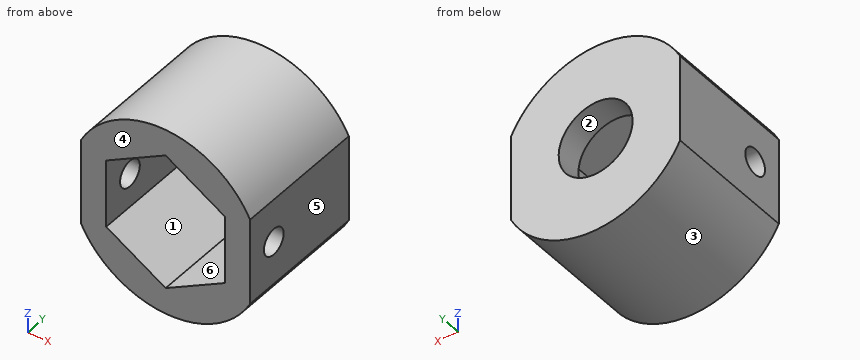
from build123d import *

# Parameters (mm, degrees)
ESBO_O9_R                   = 9
RESSALTO_EXTRUS_O1_DEPTH    = 12.5
ESBO_O12_R                  = 3.5
CORTE_EXTRUS_O9_DEPTH       = 18.839562775
CORTE_EXTRUS_O10_DEPTH      = 10
CORTE_EXTRUS_O11_DEPTH      = 18.839562775
CORTE_EXTRUS_O11_DEPTH_BACK = 18.839562775
ESBO_O14_R                  = 1.25
CORTE_EXTRUS_O12_DEPTH      = 18.83956296


with BuildPart() as part:
    # Esboço9 → Ressalto-extrusão1 (new body)
    with BuildSketch(Plane(origin=(0, 0, 0), x_dir=(1, 0, 0), z_dir=(0, 1, 0))):
        with Locations(Location((0, 0, 0), (0, 0, 270))):
            Circle(ESBO_O9_R)
    extrude(amount=RESSALTO_EXTRUS_O1_DEPTH)

    # Esboço12 → Corte-extrusão9 (cut, through all)
    with BuildSketch(Plane(origin=(0, 12.5, 0), x_dir=(1, 0, 0), z_dir=(0, 1, 0))):
        with Locations(Location((0, 0, 0), (0, 0, 270))):
            Circle(ESBO_O12_R)
    extrude(amount=-CORTE_EXTRUS_O9_DEPTH, mode=Mode.SUBTRACT)

    # Esboço13 → Corte-extrusão10 (cut)
    with BuildSketch(Plane.XZ):
        Polygon((0, 6.495190528), (-5.625, 3.247595264), (-5.625, -3.247595264), (0, -6.495190528), (5.625, -3.247595264), (5.625, 3.247595264), align=None)
    extrude(amount=-CORTE_EXTRUS_O10_DEPTH, mode=Mode.SUBTRACT)

    # Esboço14 → Corte-extrusão11 (cut, two sides: drawn at the far end of the back side and taken through both)
    with BuildSketch(Plane(origin=(0, 0, 0), x_dir=(0, 0, -1), z_dir=(1, 0, 0)).offset(-CORTE_EXTRUS_O11_DEPTH_BACK)):
        with Locations(Location((0, 3, 0), (0, 0, 270))):
            Circle(ESBO_O14_R)
    extrude(amount=CORTE_EXTRUS_O11_DEPTH + CORTE_EXTRUS_O11_DEPTH_BACK, mode=Mode.SUBTRACT)

    # Esboço15 → Corte-extrusão12 (cut, through all)
    with BuildSketch(Plane.XZ):
        with BuildLine():
            Line((-8, 4.123105626), (-8, -4.123105626))
            ThreePointArc((-8, -4.123105626), (-9, 0), (-8, 4.123105626))
        make_face()
        with BuildLine():
            Line((8, 4.123105626), (8, -4.123105626))
            ThreePointArc((8, -4.123105626), (9, 0), (8, 4.123105626))
        make_face()
    extrude(amount=-CORTE_EXTRUS_O12_DEPTH, mode=Mode.SUBTRACT)


solid = part.part
Model file for the job. Use its own axes, mm. Face numbers are marked on the shaded views. A direction names the side the tool comes from. Round coordinates to 2 decimals unless told otherwise and drop trailing zeros. Loops run counter-clockwise (first coordinate to the right, second up) from the corner with the lowest first, then second, coordinate; pieces in that order, holes last. Notation, with made-up numbers: (15.5, 29) - (48.5, 29) arc R18 cw to (48.5, 62) - close; hole circle Ø7 at (-22.75, -6.75). An arc over 180 degrees is marked (long way). Write each question's results on one line, items separated by ' | '.
(1) Saw through at C-C, the plane x = -1. List the corners of the cut face in (y, z), then the cut area to 3 significant figures.
Answer below:
outline: (0, -8.94) - (12.5, -8.94) - (12.5, -3.35) - (10, -3.35) - (10, -5.92) - (0, -5.92) - close; (0, 5.92) - (10, 5.92) - (10, 3.35) - (12.5, 3.35) - (12.5, 8.94) - (0, 8.94) - close | area: 88.5 mm^2
(2) 3-axis set-ups, long thin cutter, end or side, ignore diameter. For the marked faces 1 and 2: which of +Z, -Z, +X, -X, +Y, -Y reach the whole face in a straight line?
Answer below:
face 1: -Y | face 2: +Y, -Y
(3) Mould opens along X. For the marked faces 3, 4, 5 and 6 say: released by +X, released by -X, zero draft, split by the parting line, or undercut.
Answer below:
face 3: split by the parting line | face 4: zero draft | face 5: released by +X | face 6: undercut
(4) Saw through at D-D, the plane y = 9.25. List the corners of the cut face in (x, z) (3 decimals), then the cut area to 3 significant figures.
Answer below:
outline: (-8, -4.123) arc R9 ccw to (8, -4.123) - (8, 4.123) arc R9 ccw to (-8, 4.123) - close; hole (-5.625, -3.248) - (0, -6.495) - (5.625, -3.248) - (5.625, 3.248) - (0, 6.495) - (-5.625, 3.248) - close | area: 134 mm^2
(5) Saw through at B-B, the plane y = 3.75. List the corners of the cut face in (x, z) (3 decimals).
Answer below:
outline: (-8, -4.123) arc R9 ccw to (8, -4.123) - (8, -1) - (5.625, -1) - (5.625, -3.248) - (0, -6.495) - (-5.625, -3.248) - (-5.625, -1) - (-8, -1) - close; (-8, 1) - (-5.625, 1) - (-5.625, 3.248) - (0, 6.495) - (5.625, 3.248) - (5.625, 1) - (8, 1) - (8, 4.123) arc R9 ccw to (-8, 4.123) - close
(6) Pin check, flat tips, straight feed: pin 1 (2 mm diameter, centred on y = 3, z = 0, fed in from -X); pin 2 (5 mm diameter, centred on x = 0.5, y = 3.5, fed in from -Z); pin 3 (6 mm diameter, centred on x = -4.5, y = 10.5, fed in from +Z). Stop position of each tip, or through.
Answer below:
pin 1: passes through | pin 2: stops at z = -9 | pin 3: stops at z = 8.87
(7) Wall check: L1, parallel to X at y = 7, z = 2 (3 decimals); L2, parallel to Z at x = -1.5, y = 1.75; L3, parallel to Z at x = -7.35, y = 3. Give the ranges that are in metal, low to high.
Answer below:
L1: x = -8 to -5.625, 5.625 to 8 | L2: z = -8.87 to -5.63, 5.63 to 8.87 | L3: z = -5.19 to -1.25, 1.25 to 5.19
(8) Saw through at A-A, the plane z = 0. List the corners of the cut face in (x, y) (3 decimals), then the cut area to 3 significant figures.
Answer below:
outline: (-8, 0) - (-5.625, 0) - (-5.625, 1.75) - (-8, 1.75) - close; (-8, 4.25) - (-5.625, 4.25) - (-5.625, 10) - (-3.5, 10) - (-3.5, 12.5) - (-8, 12.5) - close; (3.5, 10) - (5.625, 10) - (5.625, 4.25) - (8, 4.25) - (8, 12.5) - (3.5, 12.5) - close; (5.625, 0) - (8, 0) - (8, 1.75) - (5.625, 1.75) - close | area: 58.1 mm^2
